Input: part model. Units: mm. Frame: model coordinates. A direction names the side the tool comes from. Round coordinates to 2 decimals unless told otherwise and drop trailing zeros. Write each loop counter-clockwise with the first axis right and the second up, starting at its lowest first coordinate (ties: lowest second). Pieces come first, ordered by that corner, then holes. Notation, with made-up numbers: M 30,34 L 65,34 A15 cw 65,52 Z; hole C -3.75,49.25 d4. An arc over 180 degrees is marked long. Use one line per item in the form item = value. Start each with the question number.
```python
from build123d import *

# Parameters (mm, degrees)
SKETCH1_W                = 370
SKETCH1_H                = 120
SKETCH1_W_2              = 350
SKETCH1_H_2              = 100
BOSS_EXTRUDE1_DEPTH      = 20
SKETCH2_R                = 3
BOSS_EXTRUDE2_DEPTH      = 30
BOSS_EXTRUDE2_DEPTH_BACK = 390
SKETCH4_W                = 2
SKETCH4_H                = 20
BOSS_EXTRUDE3_DEPTH      = 100


with BuildPart() as part:
    # Sketch1 → Boss-Extrude1 (new body)
    with BuildSketch(Plane(origin=(0, 0, 0), x_dir=(1, 0, 0), z_dir=(0, 1, 0))):
        Rectangle(SKETCH1_W, SKETCH1_H)
        Rectangle(SKETCH1_W_2, SKETCH1_H_2, mode=Mode.SUBTRACT)
    extrude(amount=BOSS_EXTRUDE1_DEPTH)

    # Sketch2 → Boss-Extrude2 (add, two sides)
    with BuildSketch(Plane.ZY.offset(185)) as boss_extrude2_sk:
        with Locations((0, 10)):
            Circle(SKETCH2_R)
    extrude(amount=BOSS_EXTRUDE2_DEPTH)
    extrude(boss_extrude2_sk.sketch, amount=-BOSS_EXTRUDE2_DEPTH_BACK)

    # Sketch4 → Boss-Extrude3 (add)
    with BuildSketch(Plane(origin=(0, 0, 50), x_dir=(-1, 0, 0), z_dir=(0, 0, -1))):
        with Locations((-125, 10)):
            Rectangle(SKETCH4_W, SKETCH4_H)
        with Locations((-75, 10)):
            Rectangle(SKETCH4_W, SKETCH4_H)
        with Locations((-25, 10)):
            Rectangle(SKETCH4_W, SKETCH4_H)
        with Locations((25, 10)):
            Rectangle(SKETCH4_W, SKETCH4_H)
        with Locations((75, 10)):
            Rectangle(SKETCH4_W, SKETCH4_H)
        with Locations((125, 10)):
            Rectangle(SKETCH4_W, SKETCH4_H)
    extrude(amount=BOSS_EXTRUDE3_DEPTH)


solid = part.part
```
Item 1: Ray query, line 1 (Z direction, x = 8.5, y = 5.25); line 2 (Z direction, x = 7, y = 7.25); line 3 (Z direction, x = 102.5, y = 8.5). Return the intervals inside material, ascending. Write a range as from..to.
Item 2: First-contact query: pin 1 (10 mm diameter, centred on y = 10.5, z = -23.5, fed in from -X); pin 2 (1.5 mm diameter, centred on y = 3.5, z = 34.5, fed in from +X); pin 3 (12 mm diameter, centred on x = -96, z = 41, fed in from -Y). Flat tips, straight axial feed; report the tip coordinate or a pass-through.
Item 3: Cut plane B-B (x = 171). Output: boundary loops of the cut face in (y, z).
Item 4: Reachability of faces 4 (the face through (-100, 10, -50)), 5 (the face through (15, 20, 54)) from +Z, -Z, +X, -X, +Y, -Y: full face, straight path, thin tool, end or side. Return the list, or none.
Item 5: Cut plane A-A (z = -13.5). Give the number of separate pieces and of enclosed holes in the cut face, plus the area to 3 significant figures.
Item 6: Draft query along X for faces 1 (the face through (76, 14, 1)), 2 (the face through (-185, 5, 1)), 3 (the face through (15, 0, 54)). Return one class per face: +X half, -X half, draft (parallel to the pull), parting line (faces both ways), or undercut.
Final values:
q1.line_1 = -60..-50, 50..60
q1.line_2 = -60..-50, -1.2..1.2, 50..60
q1.line_3 = -60..-50, -2.6..2.6, 50..60
q2.pin_1 = -185
q2.pin_2 = 185
q2.pin_3 = through
q3.outline = M 0,-60 L 20,-60 L 20,-50 L 0,-50 Z; M 0,50 L 20,50 L 20,60 L 0,60 Z; C 10,0 d6
q4.face_4 = +Y, -Y
q4.face_5 = +Z, -Z, +X, -X, +Y
q5.separate_pieces = 8
q5.enclosed_holes = 0
q5.area = 640 mm^2
q6.face_1 = undercut
q6.face_2 = -X half
q6.face_3 = draft
